Could you check a few things on this model? Use its own coordinates, in mm. A direction names the side the tool comes from. Give positions to 0.01 mm unless a question says otherwise; leave off trailing zeros. Write each loop counter-clockwise with the first axis right and the second up, starting at its lowest first coordinate (ties: lowest second). Pieces come first, ordered by that corner, then holes. Notation, with made-up numbers: (83, -10.5) -> (100, -10.5) arc R17 cw to (100, 20.5) -> close; hole circle Ø1 at (14.5, 23). An arc over 180 degrees is marked (long way). One line per question, with ' | ' between items.
from build123d import *

# Parameters (mm, degrees)
BOSS_EXTRUDE1_DEPTH      = 25
BOSS_EXTRUDE1_DEPTH_BACK = 25
SKETCH3_R                = 10
SKETCH4_R                = 16
CUT_EXTRUDE1_DEPTH       = 3.35
BOSS_EXTRUDE2_START      = 3
SKETCH5_R                = 16
SKETCH5_R_2              = 13
BOSS_EXTRUDE2_DEPTH      = 3
CHAMFER1_SIZE            = 1.523622135
CUT_EXTRUDE2_DEPTH       = 71.071392165
SKETCH11_R               = 2.6
CUT_EXTRUDE6_DEPTH       = 17.22
SKETCH12_R               = 2.6
CUT_EXTRUDE7_DEPTH       = 56.090834083


with BuildPart() as part:
    # Sketch3 → Boss-Extrude1 (new, two sides: drawn at the far end of the back side and taken through both)
    with BuildSketch(Plane(origin=(0, 0, 0), x_dir=(0, 0, -1), z_dir=(1, 0, 0)).offset(-BOSS_EXTRUDE1_DEPTH_BACK)):
        with BuildLine():
            Line((27, 0), (27, 34.44))
            Line((27, 34.44), (14.811022922, 34.44))
            ThreePointArc((14.811022922, 34.44), (0, 41), (-14.811022922, 34.44))
            Line((-14.811022922, 34.44), (-27, 34.44))
            Line((-27, 34.44), (-27, 0))
            Line((-27, 0), (27, 0))
        make_face()
        with Locations((0, 21)):
            Circle(SKETCH3_R, mode=Mode.SUBTRACT)
    extrude(amount=BOSS_EXTRUDE1_DEPTH + BOSS_EXTRUDE1_DEPTH_BACK)

    # Sketch4 → Cut-Extrude1 (cut)
    with BuildSketch(Plane(origin=(25, 0, 0), x_dir=(0, 0, -1), z_dir=(1, 0, 0))):
        with Locations((0, 21)):
            Circle(SKETCH4_R)
    cut_extrude1 = extrude(amount=-CUT_EXTRUDE1_DEPTH, mode=Mode.SUBTRACT)

    # Sketch5 → Boss-Extrude2 (add)
    with BuildSketch(Plane(origin=(21.65, 0, 0), x_dir=(0, 0, -1), z_dir=(1, 0, 0)).offset(BOSS_EXTRUDE2_START)):
        with Locations((0, 21)):
            Circle(SKETCH5_R)
        with Locations((0, 21)):
            Circle(SKETCH5_R_2, mode=Mode.SUBTRACT)
    boss_extrude2 = extrude(amount=-BOSS_EXTRUDE2_DEPTH)

    # Sketch6 → Revolve1 (revolve)
    with BuildSketch(Plane.XY, mode=Mode.PRIVATE) as revolve1_sk:
        Polygon((24.65, 31), (24.65, 31.528980942), (21.65, 32.057961884), (21.65, 31.528980942), align=None)
    revolve1 = revolve(revolve1_sk.sketch.rotate(Axis((-24.65, 21, 0), (1, 0, 0)), 90), axis=Axis((-24.65, 21, 0), (1, 0, 0)))

    # Mirror1: Cut-Extrude1, Boss-Extrude2, Revolve1 across plane
    add(cut_extrude1.mirror(Plane(origin=(0, 0, 0), x_dir=(0, 0, 1), z_dir=(1, 0, 0))), mode=Mode.SUBTRACT)
    add(boss_extrude2.mirror(Plane(origin=(0, 0, 0), x_dir=(0, 0, 1), z_dir=(1, 0, 0))))
    add(revolve1.mirror(Plane(origin=(0, 0, 0), x_dir=(0, 0, 1), z_dir=(1, 0, 0))))

    # Chamfer1
    chamfer1_edges = [part.edges().sort_by_distance(p)[0] for p in [
        (0, 34.44, 27),
        (0, 34.44, -27),
    ]]
    chamfer(chamfer1_edges, length=CHAMFER1_SIZE)

    # Sketch7 → Cut-Extrude2 (cut, through all)
    with BuildSketch(Plane(origin=(25, 0, 0), x_dir=(0, 0, -1), z_dir=(1, 0, 0))):
        Polygon((26.619094466, 5.75), (27, 5.369094466), (27, 32.916377865), (26.619094466, 33.297283399), align=None)
    extrude(amount=-CUT_EXTRUDE2_DEPTH, mode=Mode.SUBTRACT)

    # Sketch11 → Cut-Extrude6 (cut)
    with BuildSketch(Plane.XZ):
        with Locations(Location((-20, 20, 0), (0, 0, 270))):
            Circle(SKETCH11_R)
        with Locations(Location((20, 20, 0), (0, 0, 270))):
            Circle(SKETCH11_R)
        with Locations(Location((20, -20, 0), (0, 0, 270))):
            Circle(SKETCH11_R)
        with Locations(Location((-20, -20, 0), (0, 0, 270))):
            Circle(SKETCH11_R)
    extrude(amount=-CUT_EXTRUDE6_DEPTH, mode=Mode.SUBTRACT)

    # Sketch12 → Cut-Extrude7 (cut, through all)
    with BuildSketch(Plane.XZ):
        with Locations(Location((-20, 20, 0), (0, 0, 270))):
            Circle(SKETCH12_R)
        with Locations(Location((20, 20, 0), (0, 0, 270))):
            Circle(SKETCH12_R)
        with Locations(Location((20, -20, 0), (0, 0, 270))):
            Circle(SKETCH12_R)
        with Locations(Location((-20, -20, 0), (0, 0, 270))):
            Circle(SKETCH12_R)
    extrude(amount=-CUT_EXTRUDE7_DEPTH, mode=Mode.SUBTRACT)


solid = part.part
Q1. Imagine slicing it at A-A on x = 20. Please give me the cut outline in (y, z).
Answer below:
outline: (0, -27) -> (5.37, -27) -> (5.75, -26.62) -> (33.3, -26.62) -> (34.44, -25.48) -> (34.44, -22.6) -> (0, -22.6) -> close; (0, -17.4) -> (34.44, -17.4) -> (34.44, -14.81) arc R20 ccw to (34.44, 14.81) -> (34.44, 17.4) -> (0, 17.4) -> close; (0, 22.6) -> (34.44, 22.6) -> (34.44, 25.48) -> (32.92, 27) -> (0, 27) -> close; hole circle Ø20 at (21, 0)
Q2. If we mould it in two halves opening along Y, with no side actions, what happens to faces 5 (the flat face through (0, 34.44, -20)), 6 (the flat face through (0, 20, -26.619)), 7 (the cylindrical face through (-0.303, 30.915, 1.302))? For each: +Y half, -Y half, draft (parallel to the pull), parting line (faces both ways), or undercut.
Answer below:
face 5: +Y half | face 6: draft | face 7: undercut
Q3. Imagine slicing it at D-D on y = 21. Count the separate pieces of the cut face and the enclosed holes in it, and give its area (3 significant figures).
Answer below:
separate pieces: 2 | enclosed holes: 4 | area: 1,560 mm^2
Q4. If I drill on line 1 along X through (y, z) = (9, -20); line 2 along Y through (x, z) = (-24.8, 0); line 3 along Y through (x, z) = (22.9, 0), over which ranges is the centre line in solid material (lowest first)?
Answer below:
line 1: x = -25 to -22.6, -17.4 to 17.4, 22.6 to 25 | line 2: y = 0 to 5, 37 to 41 | line 3: y = 0 to 8, 10.16 to 10.69, 31.31 to 31.84, 34 to 41
Q5. Imagine slicing it at C-C on x = 7.5. Please give me the cut outline in (y, z), and give its area (3 significant figures).
Answer below:
outline: (0, -27) -> (5.37, -27) -> (5.75, -26.62) -> (33.3, -26.62) -> (34.44, -25.48) -> (34.44, -14.81) arc R20 ccw to (34.44, 14.81) -> (34.44, 25.48) -> (32.92, 27) -> (0, 27) -> close; hole circle Ø20 at (21, 0) | area: 1,670 mm^2
Q6. Imagine slicing it at B-B on z = -20. Please give me the cut outline in (x, y).
Answer below:
outline: (-25, 0) -> (-22.6, 0) -> (-22.6, 34.44) -> (-25, 34.44) -> close; (-17.4, 0) -> (17.4, 0) -> (17.4, 34.44) -> (-17.4, 34.44) -> close; (22.6, 0) -> (25, 0) -> (25, 34.44) -> (22.6, 34.44) -> close
Q7. Will these pins go through, and if not, where does the flat tip stop? pin 1 (7 mm diameter, centred on x = -20, z = 20, fed in from -Y); pin 2 (10.5 mm diameter, centred on y = 26, z = 4.5, fed in from +X); pin 3 (8 mm diameter, centred on x = 12.5, z = -7.5, fed in from +Y); pin 4 (6 mm diameter, centred on x = -15, y = 19.5, fed in from -Z).
Answer below:
pin 1: stops at y = 0 | pin 2: stops at x = 24.65 | pin 3: stops at y = 40.69 | pin 4: stops at z = -26.62
Q8. On a 3-axis mill with a long thin cutter (end or side, diameter ignored), from which of +Z, -Z, +X, -X, +Y, -Y can I reach the whole of each face in a straight line? I mean faces 1 (the flat face through (0, 0, 0)), 2 (the flat face through (-24.65, 34.1, 1.3)), 3 (the flat face through (24.65, 30, -5)), 4 (the flat face through (0, 34.44, 20)). Say none if no direction works.
Answer below:
face 1: +Z, -Z, +X, -X, -Y | face 2: -X | face 3: +X | face 4: +Z, +X, -X, +Y
